Part model, mm, in its own coordinate system. A direction names the side the tool comes from. Coordinates: 2 decimals unless noted, no trailing zeros. Write each loop counter-clockwise with the first axis right and the second up, starting at its lowest first coordinate (ties: lowest second). Pieces come first, ordered by that corner, then holes. Notation, with made-up numbers: (-11, 48) - (19, 48) arc R23 cw to (19, 82) - close; hole circle Ø6 at (73, -5.5). An arc over 180 degrees is marked (long way). Use a Markdown table: item, result.
```python
from build123d import *

# Parameters (mm, degrees)
F0_R           = 15.875
F1_DEPTH       = 25.4
F2_R           = 4.7625
F4_D           = 3.4544
F4_DEPTH       = 12.7
F6_D           = 3.4544
F6_CBORE_D     = 5.334
F6_CBORE_DEPTH = 2.54


with BuildPart() as f1:
    # F0 (on Front) → F1 (new body)
    with BuildSketch(Plane.XZ):
        with BuildLine():
            Line((-13.335, -60.325), (-13.335, -12.7))
            ThreePointArc((-13.335, -12.7), (17.097898, 6.839159), (-18.415, 0))
            Line((-18.415, 0), (-18.415, -60.325))
            Line((-18.415, -60.325), (-13.335, -60.325))
        make_face()
        Circle(F0_R, mode=Mode.SUBTRACT)
    extrude(amount=F1_DEPTH)

    # F2
    f2_edges = [f1.edges().sort_by_distance(p)[0] for p in [
        (-13.335, -12.7, -12.7),
    ]]
    fillet(f2_edges, radius=F2_R)

    # F4
    with Locations(Plane(origin=(-18.415, 0, 0), x_dir=(0, -1, 0), z_dir=(-1, 0, 0))):
        with Locations((4.572, -12.7), (20.828, -12.7)):
            Hole(F4_D / 2, depth=F4_DEPTH)

    # F6 (through all)
    with Locations(Plane.YZ.offset(-13.335)):
        with Locations((-21.59, -38.735), (-3.81, -38.735), (-21.59, -56.515), (-3.81, -56.515)):
            CounterBoreHole(F6_D / 2, F6_CBORE_D / 2, F6_CBORE_DEPTH)


solid = f1.part
```
Item 1: Drill centre lines: probe 1 along Y at (x, z) = (-12.5, -12.7); probe 2 along X at (y, z) = (-0.75, -28.5) (3 decimals); probe 3 along X at (y, z) = (-23.5, -13) (3 decimals). Where is each one in solid material? Low to high.
From the geometry:
| item | result |
|---|---|
| probe 1 | -25.4 to -22.56, -19.1 to -6.3, -2.84 to 0 |
| probe 2 | -18.415 to -13.335 |
| probe 3 | -18.415 to -9.111, 9.111 to 13.043 |
Item 2: Drop flat-ended pins along their axis: P1, Ø5, axis at y = -3.81, z = -56.515, coming from the +X side (3 decimals); P2, Ø3, axis at y = -4.572, z = -12.7, coming from the -X side; P3, Ø1, axis at y = -16.5, z = 4.5, coming from the +X side. Give the stop position or say it passes through.
From the geometry:
| item | result |
|---|---|
| P1 | x = -15.875 |
| P2 | x = 7.1 |
| P3 | x = 17.98 |
Item 3: Band-saw the part on B-B, the plane x = 0. Give the cut face in (y, z) (3 decimals).
From the geometry:
| item | result |
|---|---|
| outline | (-25.4, -18.415) - (0, -18.415) - (0, -15.875) - (-25.4, -15.875) - close; (-25.4, 15.875) - (0, 15.875) - (0, 18.415) - (-25.4, 18.415) - close |
Item 4: Which spindle directions (+Z, -Z, +X, -X, +Y, -Y) get a long thin tool onto all of the face, cutting with end or side? Do faces 1 (the face through (-13.747, -21.202, -14.386)), 2 (the face through (-14.59, -4.39, -59.12)), 3 (the face through (-17.163, -3.436, -58.201)). Say none if no direction does.
From the geometry:
| item | result |
|---|---|
| face 1 | -X |
| face 2 | +X |
| face 3 | +X, -X |
Item 5: Band-saw the part on D-D, the plane z = -12.7. Give the cut face in (x, y) (3 decimals).
From the geometry:
| item | result |
|---|---|
| outline | (-18.415, -25.4) - (-9.525, -25.4) - (-9.525, -22.555) - (-18.415, -22.555) - close; (-18.415, -19.101) - (-9.525, -19.101) - (-9.525, -6.299) - (-18.415, -6.299) - close; (-18.415, -2.845) - (-9.525, -2.845) - (-9.525, 0) - (-18.415, 0) - close; (9.525, -25.4) - (13.335, -25.4) - (13.335, 0) - (9.525, 0) - close |
Item 6: Band-saw the part on A-A, the plane z = -2. Give the cut face in (x, y) (3 decimals), then the cut area to 3 significant figures.
From the geometry:
| item | result |
|---|---|
| outline | (-18.415, -25.4) - (-15.749, -25.4) - (-15.749, 0) - (-18.415, 0) - close; (15.749, -25.4) - (18.306, -25.4) - (18.306, 0) - (15.749, 0) - close |
| area | 133 mm^2 |
Item 7: Band-saw the part on C-C, the plane y = -3.81. Count the separate pieces of the cut face and the enclosed holes in it, then the cut area to 3 significant figures.
From the geometry:
| item | result |
|---|---|
| separate pieces | 3 |
| enclosed holes | 0 |
| area | 478 mm^2 |
Item 8: Two-plate mould, pull along Y, no slides. Class faces 4 (the face through (-16, -13, -60.325)), 5 (the face through (-15.875, -2, -56)), 6 (the face through (-8, -25.4, -15)): pulls with the +Y half, pulls with the -Y half, needs draft (parallel to the pull), parting line crosses it, or undercut.
From the geometry:
| item | result |
|---|---|
| face 4 | needs draft |
| face 5 | undercut |
| face 6 | pulls with the -Y half |
